Autodesk Inventor part; units mm, degrees
ref_plane "YZ Plane" through (0, 0, 0) normal (1, 0, 0) x (0, 1, 0)
ref_plane "XZ Plane" through (0, 0, 0) normal (0, 1, 0) x (-1, 0, 0)
ref_plane "XY Plane" through (0, 0, 0) normal (0, 0, 1) x (1, 0, 0)
sketch "Boceto1" plane through (0, 0, 0) normal (1, 0, 0) x (0, 1, 0)
  point P0 (0, 0)
sketch "Boceto2" plane through (0, 0, 0) normal (0, 1, 0) x (-1, 0, 0)
  line L0 (0, 0) -> (30, 0)
  line L1 (30, 0) -> (30, -60)
  line L2 (30, -60) -> (0, -60)
  line L3 (0, -60) -> (0, 0)
  circle A0 centre (25, -5) radius 2
  line L4 (30, -30) -> (0, -30) construction
  circle A1 centre (25, -55) radius 2
  line L5 (15, 0) -> (15, -60) construction
  circle A2 centre (5, -5) radius 2
  circle A3 centre (5, -55) radius 2
  line L6 (0, -60) -> (4.6345, -112.9721)
  line L7 (0, -60) -> (53.1744, -60) construction
  line L8 (30, -60) -> (14.4189, -113.9242)
  line L9 (0, 0) -> (4.6345, 52.9721)
  line L10 (30, 0) -> (14.4189, 53.9242)
  arc A4 (14.4189, 53.9242) -> (4.6345, 52.9721) centre (9.6154, 52.5363) ccw
  arc A5 (4.6345, -112.9721) -> (14.4189, -113.9242) centre (9.6154, -112.5363) ccw
  circle A6 centre (9.6154, -112.5363) radius 2
  circle A7 centre (9.6154, 52.5363) radius 2
  line L11 (15, -60) -> (9.1311, -117.5128) construction
  line L12 (1.0267, -71.7351) -> (26.6092, -71.7351) construction
  arc A8 (21.0465, -73.7346) -> (6.3341, -72.2264) centre (13.818, -71.7351) ccw
  arc A9 (8.462, -104.6439) -> (12.3853, -105.0461) centre (10.4577, -104.5129) ccw
  line L13 (21.0465, -73.7346) -> (12.3853, -105.0461)
  line L14 (6.3018, -71.7351) -> (8.462, -104.6439)
  arc A10 (6.3341, 12.2264) -> (21.0465, 13.7346) centre (13.818, 11.7351) ccw
  arc A11 (12.3853, 45.0461) -> (8.462, 44.6439) centre (10.4577, 44.5129) ccw
  line L15 (21.0465, 13.7346) -> (12.3853, 45.0461)
  line L16 (6.3018, 11.7351) -> (8.462, 44.6439)
  point P0 (6.9725, -139.6956)
  point P1 (6.9725, 79.6956)
  dimension "d0" = 30
  dimension "d1" = 60
  dimension "d2" = 4
  dimension "d4" = 5
  dimension "d5" = 5
  dimension "d6" = 80
  dimension "d7" = 85
  dimension "d8" = 5
  dimension "d9" = 4
  dimension "d10" = 4
  dimension "d11" = 15
  dimension "d12" = 4
  dimension "d13" = 0.654
extrude "Extrusión1" add sketch "Boceto2" along normal blind 5
sketch "Boceto3" plane through (0, 5, 0) normal (0, 1, 0) x (1, 0, 0)
  point P0 (0, 0)
fillet "Empalme1" radius 10 2 edges at (-30, 2.5, 0) (-30, 2.5, -60)
The listing builds one solid part. Answer for the finished solid, in the listing's coordinates (mm). A direction names the side the tool comes from. Give positions to 0.01 mm unless a question says otherwise; leave off trailing zeros. Loops run counter-clockwise (first coordinate to the right, second up) from the corner with the lowest first, then second, coordinate; pieces in that order, holes last. Notation, with made-up numbers: (60, 8) - (110, 8) arc R26 cw to (110, 34) - close; hole circle Ø3 at (35.25, 1). An arc over 180 degrees is marked (long way). Use one line per item in the form item = value.
1. Section A-A on z = -5 is taken. Give the vertices of the cut face in (x, y), then the cut area to 3 significant figures.
Calculated:
outline = (-30, 0) - (-27, 0) - (-27, 5) - (-30, 5) - close; (-23, 0) - (-7, 0) - (-7, 5) - (-23, 5) - close; (-3, 0) - (0, 0) - (0, 5) - (-3, 5) - close
area = 110 mm^2
2. Given pin 1 Ø3.5 at (x, z) = (-25, -5) entering from +Y; pin 2 Ø1 at (x, y) = (-4.5, 4) entering from -Z; pin 3 Ø1 at (y, z) = (3.5, 29) entering from -X, each flat-ended and moving along its own axis, determine where each tip first touches the part or whether it passes through.
Calculated:
pin_1 = through
pin_2 = -114.46
pin_3 = -21.77
3. Find the intervals of material crossed by line 1 along X through (y, z) = (1.1, -6); line 2 along Z through (x, y) = (-5, 2.2); line 3 along X through (y, z) = (2.4, 10), in increasing order. Write a range as [from, to].
Calculated:
line_1 = [-30, -26.73], [-23.27, -6.73], [-3.27, 0]
line_2 = [-114.46, -57], [-53, -7], [-3, 54.46]
line_3 = [-27.11, -21.11], [-6.52, -0.87]
4. Which of the six approach directions +Z, -Z, +X, -X, +Y, -Y give full straight-line access (tool end or side, diameter ignored) to faces 1 (the face through (0, 2, -30)), 2 (the face through (-16.777, 2.465, -89.171))?
Calculated:
face_1 = +Z, -Z, +X, +Y, -Y
face_2 = +Y, -Y
5. Section D-D on z = -77 is taken. Give the vertices of the cut face in (x, y).
Calculated:
outline = (-25.09, 0) - (-20.14, 0) - (-20.14, 5) - (-25.09, 5) - close; (-6.65, 0) - (-1.49, 0) - (-1.49, 5) - (-6.65, 5) - close
6. Section C-C on y = 3.25 is taken. Count the separate pieces of the cut face and the enclosed holes in it, then the cut area to 3 significant figures.
Calculated:
separate_pieces = 1
enclosed_holes = 8
area = 3,090 mm^2
7. The mould has two halves that part along Z. Classify faces 3 (the face through (-8.141, 2.465, 51.185)), 4 (the face through (-15, 5, -29)), 5 (the face through (-22.12, 2.46, -87.27)): pulls with the +Z half, pulls with the -Z half, needs draft (parallel to the pull), parting line crosses it, or undercut.
Calculated:
face_3 = undercut
face_4 = needs draft
face_5 = pulls with the -Z half
8. Section B-B on x = -25 is taken. Give the vertices of the cut face in (y, z), then the cut area to 3 significant figures.
Calculated:
outline = (0, -77.3) - (5, -77.3) - (5, -57) - (0, -57) - close; (0, -53) - (5, -53) - (5, -7) - (0, -7) - close; (0, -3) - (5, -3) - (5, 17.3) - (0, 17.3) - close
area = 433 mm^2
